The listing builds one solid part. Answer for the finished solid, in the listing's coordinates (mm). Face numbers are marked on the shaded views. A direction names the side the tool comes from. Give positions to 0.01 mm unless a question says otherwise; leave off trailing zeros. Loops run counter-clockwise (first coordinate to the right, second up) from the corner with the lowest first, then second, coordinate; pieces in that order, holes last. Notation, with made-up numbers: (14, 89.25) - (38, 89.25) arc R32 cw to (38, 116.25) - close; hole circle Ø1 at (31, -19.75). An arc over 180 degrees is marked (long way). Write item = value, one per line. Start each with the question number.
1) The part is cut by section D-D on z = 3.25. Write down the section's boundary in (x, y).
2) Consider probe 1 along X at (y, z) = (3.25, 1.25); probe 2 along X at (y, z) = (-9.5, 1); probe 3 along Z at (x, y) = (8.5, 6.5). Determine where each line is inside the solid, lowest interval first.
3) Which of the six approach directions +Z, -Z, +X, -X, +Y, -Y give full straight-line access (tool end or side, diameter ignored) to the marked faces 1 and 2?
4) Flat-ended cylindrical pins translate along their axes: P1, Ø3, axis at x = -7.5, y = 9.5, coming from the -Z side; P2, Ø1.4, axis at y = 4.5, z = 1, coming from the -X side; P3, Ø1.8, axis at y = 13.5, z = 12, coming from the +X side; P4, Ø5, axis at x = -9.5, y = -6, coming from the +Z side. Find the tip coordinate at first contact, or state that the pin passes through.
5) The part is cut by section C-C on x = -19. Write down the section's boundary in (y, z), plus the area to 3 significant figures.
6) The part is cut by section A-A on x = -35.5. Write down the section's boundary in (y, z).
7) The part is cut by section B-B on z = 13.25. Write down the section's boundary in (x, y), plus the area to 3 significant figures.
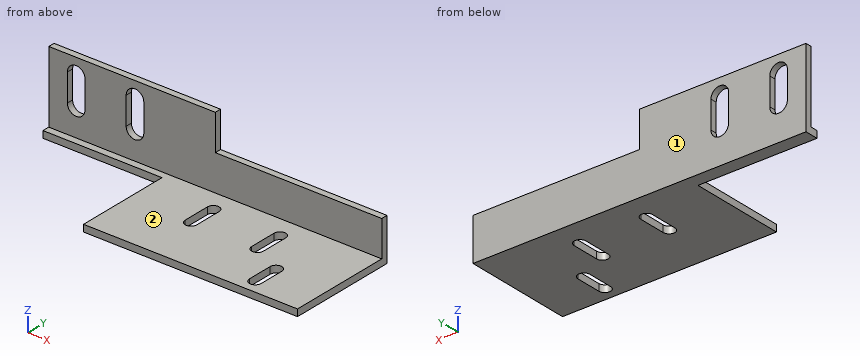
from build123d import *

# Parameters (mm, degrees)
F0_W      = 85
F0_H      = 28
F1_DEPTH  = 20
F2_W      = 26.3659512028
F2_H      = 18.2506702654
F3_DEPTH  = 121
F4_W      = 30.3753349185
F4_H      = 24.556301102
F5_DEPTH  = 25
F6_W      = 42.5
F6_H      = 9.1253351327
F7_DEPTH  = 25
F9_DEPTH  = 25
F11_DEPTH = 25


with BuildPart() as f1:
    # F0 (on Top) → F1 (new body)
    with BuildSketch(Plane.XY):
        Rectangle(F0_W, F0_H)
    extrude(amount=F1_DEPTH)

    # F2 (on face) → F3 (cut)
    with BuildSketch(Plane.YZ.offset(42.5)):
        with Locations((-0.8170243986, 10.8746648673)):
            Rectangle(F2_W, F2_H)
    extrude(amount=-F3_DEPTH, mode=Mode.SUBTRACT)

    # F4 (on face) → F5 (cut)
    with BuildSketch(Plane.XY.offset(1.7493297346)):
        with Locations((-27.3123325408, -1.721849449)):
            Rectangle(F4_W, F4_H)
    extrude(amount=-F5_DEPTH, mode=Mode.SUBTRACT)

    # F6 (on face) → F7 (cut)
    with BuildSketch(Plane.XZ.offset(-12.3659512028)):
        with Locations((21.25, 15.4373324336)):
            Rectangle(F6_W, F6_H)
    extrude(amount=-F7_DEPTH, mode=Mode.SUBTRACT)

    # F8 (on face) → F9 (cut)
    with BuildSketch(Plane.XZ.offset(-12.3659512028)):
        with BuildLine():
            ThreePointArc((-37.75, 15.8746648673), (-35.5, 13.6246648673), (-33.25, 15.8746648673))
            ThreePointArc((-33.25, 15.8746648673), (-35.5, 18.1246648673), (-37.75, 15.8746648673))
        make_face()
        with BuildLine():
            Line((-33.25, 8.8746648673), (-33.25, 15.8746648673))
            ThreePointArc((-33.25, 15.8746648673), (-35.5, 13.6246648673), (-37.75, 15.8746648673))
            Line((-37.75, 15.8746648673), (-37.75, 8.8746648673))
            ThreePointArc((-37.75, 8.8746648673), (-35.5, 11.1246648673), (-33.25, 8.8746648673))
        make_face()
        with BuildLine():
            ThreePointArc((-37.75, 8.8746648673), (-35.5, 6.6246648673), (-33.25, 8.8746648673))
            ThreePointArc((-33.25, 8.8746648673), (-35.5, 11.1246648673), (-37.75, 8.8746648673))
        make_face()
        with BuildLine():
            ThreePointArc((-22.75, 8.8746648673), (-20.5, 6.6246648673), (-18.25, 8.8746648673))
            ThreePointArc((-18.25, 8.8746648673), (-20.5, 11.1246648673), (-22.75, 8.8746648673))
        make_face()
        with BuildLine():
            ThreePointArc((-22.75, 8.8746648673), (-20.5, 11.1246648673), (-18.25, 8.8746648673))
            Line((-18.25, 8.8746648673), (-18.25, 15.8746648673))
            ThreePointArc((-18.25, 15.8746648673), (-20.5, 13.6246648673), (-22.75, 15.8746648673))
            Line((-22.75, 15.8746648673), (-22.75, 8.8746648673))
        make_face()
        with BuildLine():
            ThreePointArc((-22.75, 15.8746648673), (-20.5, 13.6246648673), (-18.25, 15.8746648673))
            ThreePointArc((-18.25, 15.8746648673), (-20.5, 18.1246648673), (-22.75, 15.8746648673))
        make_face()
    extrude(amount=-F9_DEPTH, mode=Mode.SUBTRACT)

    # F10 (on face) → F11 (cut)
    with BuildSketch(Plane.XY.offset(1.7493297346)):
        with BuildLine():
            ThreePointArc((2.3753349185, 7), (3.8753349185, 5.5), (5.3753349185, 7))
            ThreePointArc((5.3753349185, 7), (3.8753349185, 8.5), (2.3753349185, 7))
        make_face()
        with BuildLine():
            Line((5.3753349185, 0), (5.3753349185, 7))
            ThreePointArc((5.3753349185, 7), (3.8753349185, 5.5), (2.3753349185, 7))
            Line((2.3753349185, 7), (2.3753349185, 0))
            ThreePointArc((2.3753349185, 0), (3.8753349185, 1.5), (5.3753349185, 0))
        make_face()
        with BuildLine():
            ThreePointArc((2.3753349185, 0), (3.8753349185, -1.5), (5.3753349185, 0))
            ThreePointArc((5.3753349185, 0), (3.8753349185, 1.5), (2.3753349185, 0))
        make_face()
        with BuildLine():
            ThreePointArc((19.3753349185, 7), (20.8753349185, 5.5), (22.3753349185, 7))
            ThreePointArc((22.3753349185, 7), (20.8753349185, 8.5), (19.3753349185, 7))
        make_face()
        with BuildLine():
            Line((22.3753349185, 0), (22.3753349185, 7))
            ThreePointArc((22.3753349185, 7), (20.8753349185, 5.5), (19.3753349185, 7))
            Line((19.3753349185, 7), (19.3753349185, 0))
            ThreePointArc((19.3753349185, 0), (20.8753349185, 1.5), (22.3753349185, 0))
        make_face()
        with BuildLine():
            ThreePointArc((19.3753349185, 0), (20.8753349185, -1.5), (22.3753349185, 0))
            ThreePointArc((22.3753349185, 0), (20.8753349185, 1.5), (19.3753349185, 0))
        make_face()
        with BuildLine():
            ThreePointArc((27.3753349185, -4.0281792737), (28.8753349185, -5.5281792737), (30.3753349185, -4.0281792737))
            ThreePointArc((30.3753349185, -4.0281792737), (28.8753349185, -2.5281792737), (27.3753349185, -4.0281792737))
        make_face()
        with BuildLine():
            Line((30.3753349185, -10.5132134631), (30.3753349185, -4.0281792737))
            ThreePointArc((30.3753349185, -4.0281792737), (28.8753349185, -5.5281792737), (27.3753349185, -4.0281792737))
            Line((27.3753349185, -4.0281792737), (27.3753349185, -10.5132134631))
            ThreePointArc((27.3753349185, -10.5132134631), (28.8753349185, -9.0132134631), (30.3753349185, -10.5132134631))
        make_face()
        with BuildLine():
            ThreePointArc((27.3753349185, -10.5132134631), (28.8753349185, -12.0132134631), (30.3753349185, -10.5132134631))
            ThreePointArc((30.3753349185, -10.5132134631), (28.8753349185, -9.0132134631), (27.3753349185, -10.5132134631))
        make_face()
    extrude(amount=-F11_DEPTH, mode=Mode.SUBTRACT)


solid = f1.part
Answer below:
q1.outline = (-42.5, 12.37) - (42.5, 12.37) - (42.5, 14) - (-42.5, 14) - close
q2.probe_1 = -12.12 to 2.38, 5.38 to 19.38, 22.38 to 42.5
q2.probe_2 = -12.12 to 27.38, 30.38 to 42.5
q2.probe_3 = 0 to 1.75
q3.face_1 = +Z, -Z, +X, -X, +Y
q3.face_2 = +Z, +X, -X, -Y
q4.P1 = 0
q4.P2 = -12.12
q4.P3 = 0
q4.P4 = 1.75
q5.outline = (10.56, 0) - (14, 0) - (14, 7.2) - (12.37, 7.2) - (12.37, 1.75) - (10.56, 1.75) - close; (12.37, 17.55) - (14, 17.55) - (14, 20) - (12.37, 20) - close
q5.area = 18.9 mm2
q6.outline = (10.56, 0) - (14, 0) - (14, 6.62) - (12.37, 6.62) - (12.37, 1.75) - (10.56, 1.75) - close; (12.37, 18.12) - (14, 18.12) - (14, 20) - (12.37, 20) - close
q7.outline = (-42.5, 12.37) - (-37.75, 12.37) - (-37.75, 14) - (-42.5, 14) - close; (-33.25, 12.37) - (-22.75, 12.37) - (-22.75, 14) - (-33.25, 14) - close; (-18.25, 12.37) - (0, 12.37) - (0, 14) - (-18.25, 14) - close
q7.area = 54.7 mm2
